Autodesk Inventor part; units mm, degrees
ref_plane "YZ Plane" through (0, 0, 0) normal (1, 0, 0) x (0, 1, 0)
ref_plane "XZ Plane" through (0, 0, 0) normal (0, 1, 0) x (-1, 0, 0)
ref_plane "XY Plane" through (0, 0, 0) normal (0, 0, 1) x (1, 0, 0)
sketch "Sketch1" plane through (0, 0, 0) normal (0, 0, 1) x (1, 0, 0)
  line L0 (-6, -5) -> (6, -5)
  line L1 (6, -5) -> (6, 5)
  line L2 (6, 5) -> (-6, 5)
  line L3 (-6, 5) -> (-6, -5)
  line L4 (-6, -5) -> (6, 5) construction
  line L5 (6, -5) -> (-6, 5) construction
  point P0 (0, 0)
  dimension "d0" = 12
  dimension "d1" = 10
extrude "Extrusion1" add sketch "Sketch1" along normal mid plane 26
sketch "Sketch2" plane through (0, 0, 13) normal (0, 0, 1) x (1, 0, 0)
  circle A0 centre (0, 0) radius 1.5
  circle A1 centre (0, 0) radius 2
  dimension "d4" = 3
  dimension "d12" = 4
extrude "Extrusion2" add sketch "Sketch2" along normal blind 55 contours A0
fillet "Fillet1" radius 1 4 edges at (6, 5, 0) (-6, 5, 0) (6, -5, 0) (-6, -5, 0)
sketch "Sketch3" plane through (0, 0, -13) normal (0, 0, -1) x (-1, 0, 0)
  arc A0 (5, -5) -> (6, -4) centre (5, -4) ccw
  line L0 (6, -4) -> (6, 4)
  arc A1 (6, 4) -> (5, 5) centre (5, 4) ccw
  line L1 (5, 5) -> (-5, 5)
  arc A2 (-5, 5) -> (-6, 4) centre (-5, 4) ccw
  line L2 (-6, 4) -> (-6, -4)
  arc A3 (-6, -4) -> (-5, -5) centre (-5, -4) ccw
  line L3 (-5, -5) -> (5, -5)
  circle A4 centre (0, 0) radius 6
  point P0 (3.3166, 5)
  point P1 (6, 0)
  point P2 (3.3166, -5)
  point P3 (-3.3166, -5)
  point P4 (-6, 0)
  point P5 (-3.3166, 5)
  dimension "d8" = 12
extrude "Extrusion3" cut sketch "Sketch3" against normal blind 17 contours L3 A4 L0 A0 | A4 L1 A1 L0 | L3 A3 L2 A4 | L2 A2 L1 A4
fillet "Fillet2" radius 0.5 4 edges at (-3.3166, -5, -4.5) (3.3166, -5, -4.5) (-3.3166, 5, -4.5) (3.3166, 5, -4.5)
extrude "Extrusion4" add sketch "Sketch2" along normal blind 0.5
chamfer "Chamfer1" distance 0.25 angle 45 1 edges at (-1.5, 0, 68)
properties part number "DC Motor"
Read the model definition and answer for the solid it produces. Units are mm, in the model's axes. A direction names the side the tool comes from. Give positions to 0.01 mm unless a question says otherwise; leave off trailing zeros. Order: outer loops, then holes, each group sorted by start corner. A loop starts at its lowest first (then second) coordinate and runs counter-clockwise, first axis right, second up. Notation, with made-up numbers: (-2, 7.25) -> (23, 7.25) arc R12 ccw to (23, 13.25) -> close; hole circle Ø1 at (-18, 73.5). An arc over 180 degrees is marked (long way). Write item = value, one per line.
1. A cutting plane is placed at B-B, the plane y = 3. Write down the section's boundary in (x, z).
Numbers:
outline = (-6, 4) -> (-5.2, 4) -> (-5.2, -13) -> (5.2, -13) -> (5.2, 4) -> (6, 4) -> (6, 13) -> (-6, 13) -> close
2. Straight lines are drawn through the part: line 1 along Z through (x, y) = (-4.75, -2.5); line 2 along Z through (x, y) = (5.5, 3.75); line 3 along X through (y, z) = (0.75, 47.5). For each, find the intervals that lie inside material, in ascending order.
Numbers:
line_1 = -13 to 13
line_2 = 4 to 13
line_3 = -1.3 to 1.3
3. For faces 1 (the face through (-6, 0, -5)), 2 (the face through (-5, -4, 4)), 3 (the face through (6, 0, -5)), 4 (the face through (-0.1, 2.3, 13)), determine the directions among +Z, -Z, +X, -X, +Y, -Y from which every point of the face is accessible in a straight line to the end or side of a thin tool.
Numbers:
face_1 = -Z, -X
face_2 = -Z, -X, -Y
face_3 = -Z, +X
face_4 = +Z
4. Given pin 1 (4 mm diameter, centred on x = 4, z = 46, fed in from -Y); pin 2 (2 mm diameter, centred on x = -1.5, z = 30, fed in from +Y); pin 3 (3 mm diameter, centred on y = 0.5, z = 41, fed in from +X); pin 4 (1 mm diameter, centred on x = -4.5, y = -0.5, fed in from +Z), each flat-ended and moving along its own axis, determine where each tip first touches the part or whether it passes through.
Numbers:
pin_1 = through
pin_2 = 1.41
pin_3 = 1.5
pin_4 = 13
5. A cutting plane is placed at A-A, the plane x = 0. Write down the section's boundary in (y, z), and give its area (3 significant figures).
Numbers:
outline = (-5, -13) -> (5, -13) -> (5, 13) -> (2, 13) -> (2, 13.5) -> (1.5, 13.5) -> (1.5, 67.75) -> (1.25, 68) -> (-1.25, 68) -> (-1.5, 67.75) -> (-1.5, 13.5) -> (-2, 13.5) -> (-2, 13) -> (-5, 13) -> close
area = 425 mm²
6. A cutting plane is placed at D-D, the plane x = 4.25. Write down the section's boundary in (y, z).
Numbers:
outline = (-5, 4) -> (-4.24, 4) -> (-4.24, -13) -> (4.24, -13) -> (4.24, 4) -> (5, 4) -> (5, 13) -> (-5, 13) -> close
7. A cutting plane is placed at C-C, the plane z = 58. Write down the section's boundary in (x, y), and give its area (3 significant figures).
Numbers:
outline = circle Ø3 at (0, 0)
area = 7.07 mm²
